Job drawing, mm, ordinate dimensions from the low corner. One solid piece. A direction names the side the tool comes from. Give positions to 0.01 mm unless a question says otherwise; leave off trailing zeros. Write each loop counter-clockwise with the first axis right and the second up, starting at its lowest first coordinate (ties: lowest second). Pieces come first, ordered by that corner, then holes. Notation, with made-up numbers: M 45,8 L 85,8 A28 cw 85,29 Z; hole C 33.25,57 d9. An arc over 180 degrees is marked long. Use CSV: the item, a comma, the result in double quotes. Start each with the question number.
Item 1: Mould opens along Y. For the marked faces 1, 2 and 3 say: released by +Y, released by -Y, zero draft, split by the parting line, or undercut.
Item 2: Cut at D-D (y = 47). List the corners of the cut face in (x, z) (3 decimals), then the cut area to 3 significant figures.
Item 3: Pin check, flat tips, straight feed: pin 1 (4 mm diameter, centred on x = 55, z = 19, fed in from -Y); pin 2 (12 mm diameter, centred on x = 45.5, z = 19, fed in from -Y); pin 3 (8 mm diameter, centred on y = 35.5, z = 4.5, fed in from -X); pin 4 (12 mm diameter, centred on x = 29.5, y = 18.5, fed in from -Z) (3 decimals). Stop position of each tip, or through.
Item 4: Cut at C-C (z = 8). List the corners of the cut face in (x, y).
Item 5: Drill centre lines: line 1 (Y direction, x = 38.1, z = 26); line 2 (Y direction, x = 38, z = 19); line 3 (Z direction, x = 71, y = 41) (3 decimals). Where is each one in solid material? Low to high. Write a range as [from, to].
Item 6: Cut at A-A (y = 38.1). List the corners of the cut face in (x, z) (3 decimals).
Item 7: Which spindle directions (+Z, -Z, +X, -X, +Y, -Y) get a long thin tool onto all of the face, cutting with end or side? Do the marked faces 4 and 5. Say none if no direction does.
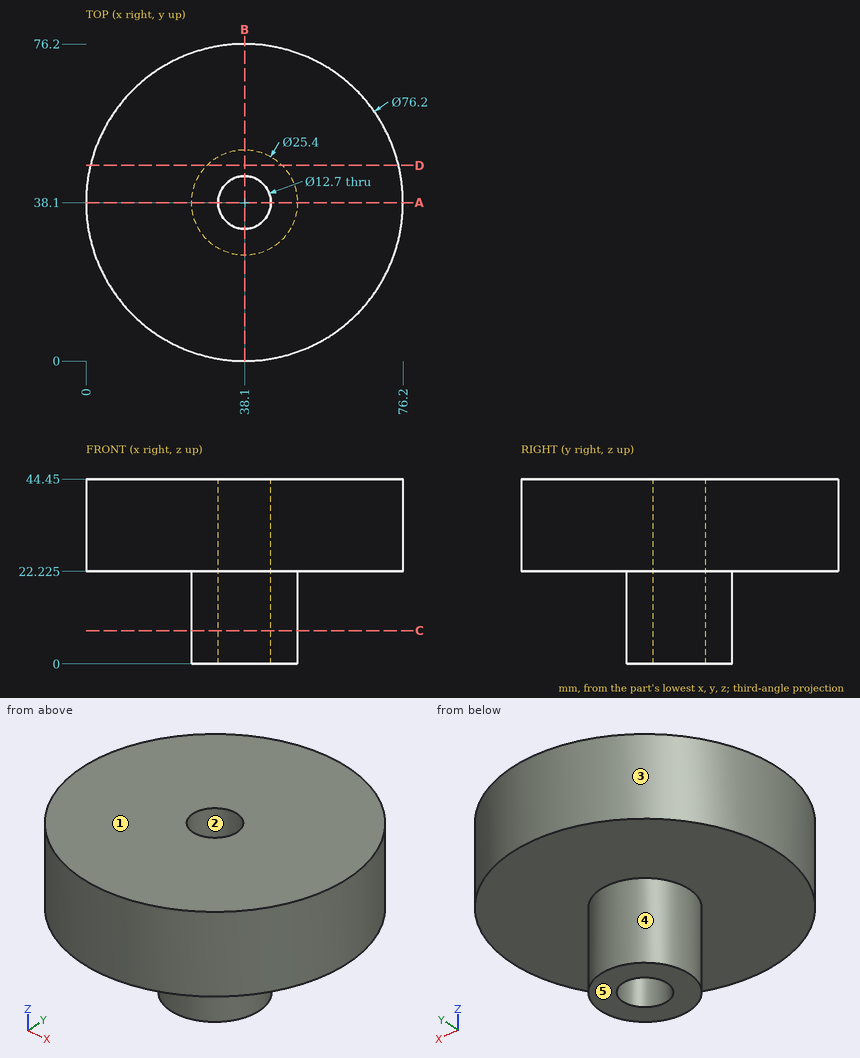
Worked answers:
1,face 1,"zero draft"
1,face 2,"undercut"
1,face 3,"split by the parting line"
2,outline,"M 1.054,22.225 L 29.04,22.225 L 29.04,0 L 47.16,0 L 47.16,22.225 L 75.146,22.225 L 75.146,44.45 L 1.054,44.45 Z"
2,area,"2,050 mm^2"
3,pin 1,"passes through"
3,pin 2,"stops at y = 0.07"
3,pin 3,"stops at x = 25.4"
3,pin 4,"stops at z = 22.225"
4,outline,"C 38.1,38.1 d25.4; hole C 38.1,38.1 d12.7"
5,line 1,"y = [0, 31.75], [44.45, 76.2]"
5,line 2,"y = [25.4, 31.75], [44.45, 50.8]"
5,line 3,"z = [22.225, 44.45]"
6,outline,"M 0,22.225 L 25.4,22.225 L 25.4,0 L 31.75,0 L 31.75,44.45 L 0,44.45 Z; M 44.45,0 L 50.8,0 L 50.8,22.225 L 76.2,22.225 L 76.2,44.45 L 44.45,44.45 Z"
7,face 4,"-Z"
7,face 5,"-Z, +X, -X, +Y, -Y"
